Geometry check sheet. Reference: the model listing, model coordinates, mm. A direction names the side the tool comes from. Give positions to 0.01 mm unless a question says otherwise; leave off trailing zeros. Loops run counter-clockwise (first coordinate to the right, second up) from the corner with the lowest first, then second, coordinate; pieces in that order, holes last.
1. Cross-section at A-A, the plane y = 0. Record the cut outline in (x, z).
2. Cross-section at C-C, the plane x = -1.35. Record the cut outline in (y, z).
3. Release check for a two-part mould opening along Y. For faces 1 (the flat face through (-2.585, -3.96, -0.07)), 2 (the flat face through (-2, 0, 5)), 3 (the cylindrical face through (-2.03, -1.64, -1.26)), 4 (the flat face through (-2.546, 3.988, -0.07)) record: +Y half, -Y half, draft (parallel to the pull), parting line (faces both ways), or undercut.
4. Cross-section at B-B, the plane z = 0. Record the cut outline in (x, y).
5. Material ranges on L1, parallel to Z at x = -1.05, y = 0; L2, parallel to Y at x = -3.45, z = -1.75 (3 decimals); L3, parallel to Y at x = -1.1, z = -3.5, recorded low to high.
6. Cross-section at D-D, the plane x = -2.9. Record the cut outline in (y, z).
7. Tool access check on faces 5 (the flat face through (-4.1, -2.4, -1.2)), 6 (the flat face through (-0.8, -4, 0)), 7 (the flat face through (-0.8, 4, 0)). Record the directions out of +Z, -Z, +X, -X, +Y, -Y that give a thin tool (end or side, any length) a straight path to the whole face; none if there is none.
8. Go/stop test with a flat-tipped pin: pin 1 Ø0.6 at (y, z) = (-4, -1.5) entering from +X. Record where the tip stops, or that it passes through.
Autodesk Inventor part; units mm, degrees
ref_plane "nut_XY" through (0, 0, 0) normal (1, 0, 0) x (0, 0, -1)
ref_plane "nut_YZ" through (0, 0, 0) normal (0, 0, -1) x (0, 1, 0)
ref_plane "nut_ZX" through (0, 0, 0) normal (0, 1, 0) x (1, 0, 0)
sketch "Sketch_2" plane through (0, 0, 0) normal (0, 0, 1) x (1, 0, 0)
  arc A0 (-4.1, -2.7438) -> (-3.972, -2.9896) centre (-3.8, -2.7438) ccw
  line L0 (-3.972, -2.9896) -> (-1.1589, -4.9588)
  arc A1 (-1.1589, -4.9588) -> (-0.8, -4.7719) centre (-1.0281, -4.7719) ccw
  line L1 (-0.8, -4.7719) -> (-0.8, -2.9)
  line L2 (-0.8, -2.9) -> (-0.2, -2.9)
  arc A2 (-0.2, -2.9) -> (0, -2.7) centre (-0.2, -2.7) ccw
  line L3 (0, -2.7) -> (0, 2.7)
  arc A3 (0, 2.7) -> (-0.2, 2.9) centre (-0.2, 2.7) ccw
  line L4 (-0.2, 2.9) -> (-0.8, 2.9)
  line L5 (-0.8, 2.9) -> (-0.8, 4.7719)
  arc A4 (-0.8, 4.7719) -> (-1.1589, 4.9588) centre (-1.0281, 4.7719) ccw
  line L6 (-1.1589, 4.9588) -> (-3.972, 2.9896)
  arc A5 (-3.972, 2.9896) -> (-4.1, 2.7438) centre (-3.8, 2.7438) ccw
  line L7 (-4.1, 2.7438) -> (-4.1, -2.7438)
extrude "Extrusion1" add sketch "Sketch_2" along normal mid plane 10
sketch "Sketch_5" plane through (0, 0, 0) normal (0, 0, 1) x (1, 0, 0)
  line L0 (0, 0) -> (-4.1, 0)
  line L1 (-4.1, 0) -> (-4.1, 2.5)
  line L2 (-4.1, 2.5) -> (-3.667, 2.067)
  line L3 (-3.667, 2.067) -> (-0.433, 2.067)
  line L4 (-0.433, 2.067) -> (0, 2.5)
  line L5 (0, 2.5) -> (0, 0)
  line L6 (0, 0) -> (-4.1, 0)
revolve "Revolution1" cut sketch "Sketch_5" angle 360 about axis through (0, 0, 0) along (1, 0, 0)
thread "Thread1"
ref_plane "nut_XY" through (0, 0, 0) normal (1, 0, 0) x (0, 0, -1)
ref_plane "nut_YZ" through (0, 0, 0) normal (0, 0, -1) x (0, 1, 0)
ref_plane "nut_ZX" through (0, 0, 0) normal (0, 1, 0) x (1, 0, 0)
ref_plane "to_bolt_XY" through (-4.1, 0, 0) normal (1, 0, 0) x (0, 0, -1)
ref_plane "to_bolt_YZ" through (-4.1, 0, 0) normal (0, 0, -1) x (0, 1, 0)
ref_plane "to_bolt_ZX" through (-4.1, 0, 0) normal (0, 1, 0) x (1, 0, 0)
ref_plane "to_frames_XY" through (-0.8, 0, 0) normal (1, 0, 0) x (0, 0, -1)
ref_plane "to_frames_YZ" through (-0.8, 0, 0) normal (0, 0, -1) x (0, 1, 0)
ref_plane "to_frames_ZX" through (-0.8, 0, 0) normal (0, 1, 0) x (1, 0, 0)
ref_plane "to_lane_XY" through (0, 0, 0) normal (0, 0, 1) x (1, 0, 0)
ref_plane "to_lane_YZ" through (0, 0, 0) normal (1, 0, 0) x (0, 1, 0)
ref_plane "to_lane_ZX" through (0, 0, 0) normal (0, 1, 0) x (0, 0, 1)
properties part number "HNTTSS5-5"
Result:
1. outline: (-4.1, -5) - (0, -5) - (0, -2.5) - (-0.43, -2.07) - (-3.67, -2.07) - (-4.1, -2.5) - close; (-4.1, 2.5) - (-3.67, 2.07) - (-0.43, 2.07) - (0, 2.5) - (0, 5) - (-4.1, 5) - close
2. outline: (-4.83, -5) - (4.83, -5) - (4.83, 5) - (-4.83, 5) - close; hole circle Ø4.13 at (0, 0)
3. face 1: -Y half
3. face 2: draft
3. face 3: undercut
3. face 4: +Y half
4. outline: (-4.1, -2.74) arc R0.3 ccw to (-3.97, -2.99) - (-1.16, -4.96) arc R0.23 ccw to (-0.8, -4.77) - (-0.8, -2.9) - (-0.2, -2.9) arc R0.2 ccw to (0, -2.7) - (0, -2.5) - (-0.43, -2.07) - (-3.67, -2.07) - (-4.1, -2.5) - close; (-4.1, 2.5) - (-3.67, 2.07) - (-0.43, 2.07) - (0, 2.5) - (0, 2.7) arc R0.2 ccw to (-0.2, 2.9) - (-0.8, 2.9) - (-0.8, 4.77) arc R0.23 ccw to (-1.16, 4.96) - (-3.97, 2.99) arc R0.3 ccw to (-4.1, 2.74) - close
5. L1: z = -5 to -2.07, 2.07 to 5
5. L2: y = -3.355 to -1.1, 1.1 to 3.355
5. L3: y = -4.99 to 4.99
6. outline: (-3.74, -5) - (3.74, -5) - (3.74, 5) - (-3.74, 5) - close; hole circle Ø4.13 at (0, 0)
7. face 5: +Z, -Z, -X, +Y, -Y
7. face 6: +Z, -Z, +X, -Y
7. face 7: +Z, -Z, +X, +Y
8. pin 1: stops at x = -0.8
